Model file for the job. Use its own axes, mm. Face numbers are marked on the shaded views. A direction names the side the tool comes from. Give positions to 0.01 mm unless a question says otherwise; leave off trailing zeros. Order: outer loops, then holes, each group sorted by start corner. A loop starts at its lowest first (then second) coordinate and runs counter-clockwise, first axis right, second up. Notation, with made-up numbers: (-5, 44.25) -> (36, 44.25) arc R9 ccw to (36, 54.25) -> close; hole circle Ø7 at (81.25, -28). An arc over 180 degrees is marked (long way). Answer in a Markdown table with one row per item. Add a question column.
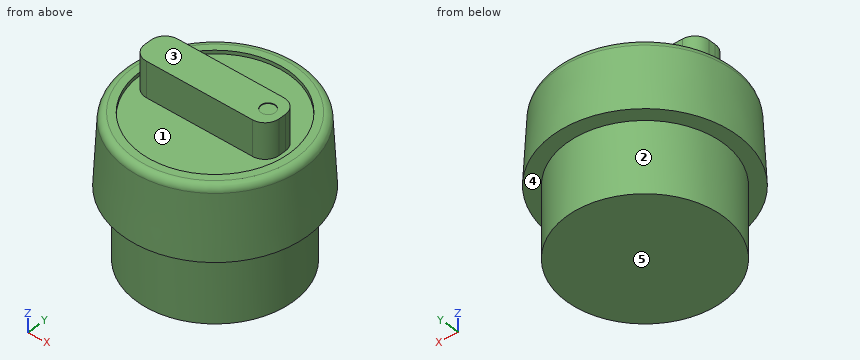
from build123d import *

# Parameters (mm, degrees)
SKETCH_1_R          = 11
EXTRUDE_1_DEPTH     = 10
SKETCH_2_R          = 13
EXTRUDE_2_DEPTH     = 10
EXTRUDE_2_TAPER     = 3
FILLET_1_R          = 1
SKETCH_3_R          = 10.5
CUT_EXTRUDE_1_DEPTH = 0.5
SKETCH_4_W          = 19
SKETCH_4_H          = 5
EXTRUDE_4_DEPTH     = 5
FILLET_3_R          = 2
SKETCH_5_R          = 1
CUT_EXTRUDE_2_DEPTH = 0.1


with BuildPart() as part:
    # 草图1 → 凸台-拉伸1 (new body)
    with BuildSketch(Plane.XY):
        Circle(SKETCH_1_R)
    extrude(amount=EXTRUDE_1_DEPTH)

    # 草图2 → 凸台-拉伸2 (add)
    with BuildSketch(Plane.XY.offset(10)):
        Circle(SKETCH_2_R)
    extrude(amount=EXTRUDE_2_DEPTH, taper=EXTRUDE_2_TAPER)

    # 圆角1
    fillet_1_edges = [part.edges().sort_by_distance(p)[0] for p in [
        (-12.475922207, 0, 20),
    ]]
    fillet(fillet_1_edges, radius=FILLET_1_R)

    # 草图3 → 切除-拉伸1 (cut)
    with BuildSketch(Plane.XY.offset(20)):
        Circle(SKETCH_3_R)
    extrude(amount=-CUT_EXTRUDE_1_DEPTH, mode=Mode.SUBTRACT)

    # 草图4 → 凸台-拉伸4 (add)
    with BuildSketch(Plane.XY.offset(19.5)):
        Rectangle(SKETCH_4_W, SKETCH_4_H)
    extrude(amount=EXTRUDE_4_DEPTH)

    # 圆角3
    fillet_3_edges = [part.edges().sort_by_distance(p)[0] for p in [
        (-9.5, 2.5, 22),
        (-9.5, -2.5, 22),
        (9.5, -2.5, 22),
        (9.5, 2.5, 22),
    ]]
    fillet(fillet_3_edges, radius=FILLET_3_R)

    # 草图5 → 切除-拉伸2 (cut)
    with BuildSketch(Plane.XY.offset(24.5)):
        with Locations((7.5, 0)):
            Circle(SKETCH_5_R)
    extrude(amount=-CUT_EXTRUDE_2_DEPTH, mode=Mode.SUBTRACT)


solid = part.part
Item 1: Saw through at B-B on y = 0. List the corners of the cut face in (x, z).
Item 2: Saw through at C-C on z = 5. List the corners of the cut face in (x, y).
Item 3: Saw through at D-D on z = 18.25. List the corners of the cut face in (x, y), plus the area to 3 significant figures.
Item 4: Two-plate mould, pull along Y, no slides. Class the marked faces 1, 2 and 3: pulls with the +Y half, pulls with the -Y half, needs draft (parallel to the pull), parting line crosses it, or undercut.
Item 5: Wall check: line 1 (Y direction, x = 0, z = 19.7); line 2 (Y direction, x = 7.5, z = 24.45); line 3 (Y direction, x = 0, z = 19.8). Give the ranges that are in metal, low to high.
Item 6: Pin check, flat tips, straight feed: pin 1 Ø1 at (y, z) = (6, 16) entering from -X; pin 2 Ø1.5 at (x, z) = (-8, 6) entering from +Y; pin 3 Ø8 at (y, z) = (-8.5, 7) entering from -X. Stop position of each tip, or through.
Item 7: Which spindle directions (+Z, -Z, +X, -X, +Y, -Y) get a long thin tool onto all of the face, cutting with end or side? Do the marked faces 4 and 5. Say none if no direction does.
Item 8: Saw through at A-A on x = 0. List the corners of the cut face in (y, z), plus the area to 3 significant figures.
Evaluation:
| question | item | result |
|---|---|---|
| 1 | outline | (-13, 10) -> (-11, 10) -> (-11, 0) -> (11, 0) -> (11, 10) -> (13, 10) -> (12.53, 19.05) arc R1 ccw to (11.53, 20) -> (10.5, 20) -> (10.5, 19.5) -> (9.5, 19.5) -> (9.5, 24.5) -> (8.5, 24.5) -> (8.5, 24.4) -> (6.5, 24.4) -> (6.5, 24.5) -> (-9.5, 24.5) -> (-9.5, 19.5) -> (-10.5, 19.5) -> (-10.5, 20) -> (-11.53, 20) arc R1 ccw to (-12.53, 19.05) -> close |
| 2 | outline | circle Ø22 at (0, 0) |
| 3 | outline | circle Ø25.14 at (0, 0) |
| 3 | area | 496 mm2 |
| 4 | face 1 | undercut |
| 4 | face 2 | parting line crosses it |
| 4 | face 3 | needs draft |
| 5 | line 1 | y = -12.24 to -10.5, -2.5 to 2.5, 10.5 to 12.24 |
| 5 | line 2 | y = -2.5 to -1, 1 to 2.5 |
| 5 | line 3 | y = -12.13 to -10.5, -2.5 to 2.5, 10.5 to 12.13 |
| 6 | pin 1 | stops at x = -11.43 |
| 6 | pin 2 | stops at y = 8.27 |
| 6 | pin 3 | stops at x = -11.61 |
| 7 | face 4 | -Z |
| 7 | face 5 | -Z, +X, -X, +Y, -Y |
| 8 | outline | (-13, 10) -> (-11, 10) -> (-11, 0) -> (11, 0) -> (11, 10) -> (13, 10) -> (12.53, 19.05) arc R1 ccw to (11.53, 20) -> (10.5, 20) -> (10.5, 19.5) -> (2.5, 19.5) -> (2.5, 24.5) -> (-2.5, 24.5) -> (-2.5, 19.5) -> (-10.5, 19.5) -> (-10.5, 20) -> (-11.53, 20) arc R1 ccw to (-12.53, 19.05) -> close |
| 8 | area | 489 mm2 |
